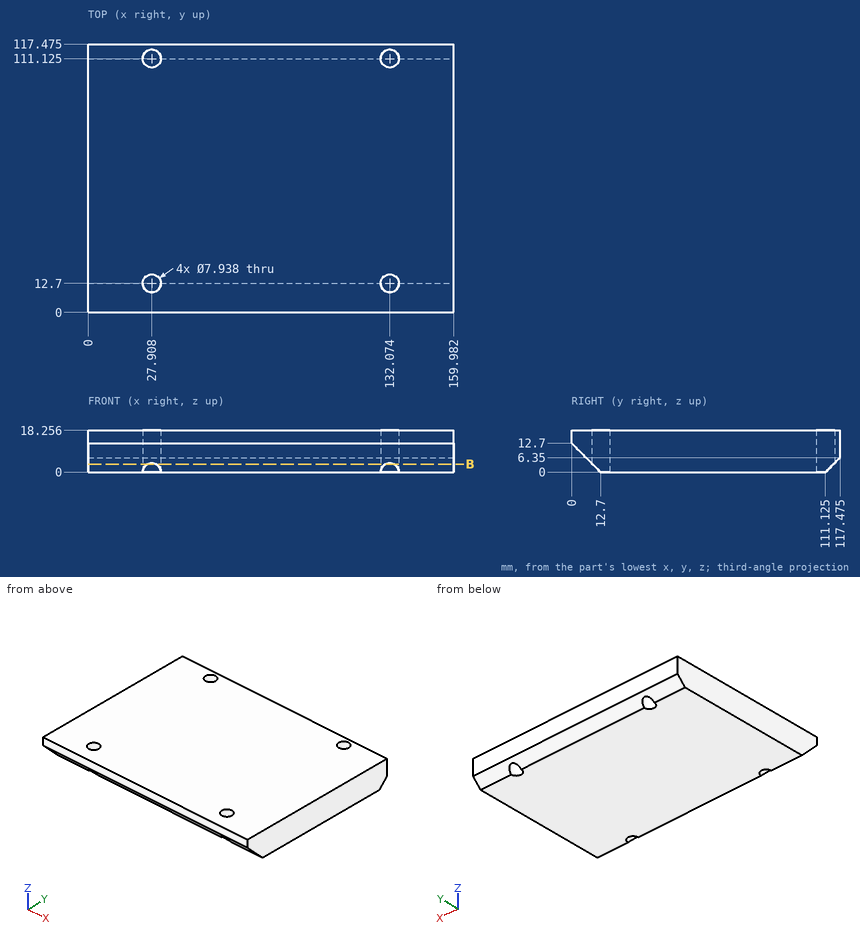
For this review, use the dimensioned drawing (mm, ordinates from the lowest corner) and the shaded views. Give positions to 0.01 mm unless a question says otherwise; leave off trailing zeros. Write each loop counter-clockwise with the first axis right and the second up, starting at its lowest first coordinate (ties: lowest second). Pieces come first, ordered by that corner, then holes.
(1) To check wall thickness, follow L1, parallel to Z at x = 15, y = 5 (1 decimal); L2, parallel to Y at x = 64.5, z = 7.5 (1 decimal); L3, parallel to Y at x = 58, z = 5 (1 decimal). State the ranges of each line that lie inside material, in increasing order.
(2) Consider section B-B, the plane z = 3.5. Give the boundary of the cut face in (x, y) (1 decimal).
(3) For P1, Ø1, axis at x = 45, z = 5, coming from the -Y side; P2, Ø3, axis at x = 125.5, z = 10, coming from the -Y side, all flat-tipped, find the tip position at first contact; note any pin that passes through.
Returned:
1. L1: z = 7.7 to 18.3
1. L2: y = 5.2 to 117.5
1. L3: y = 7.7 to 116.1
2. outline: (0, 9.2) - (26, 9.2) arc R4 cw (long way) to (29.8, 9.2) - (130.2, 9.2) arc R4 cw (long way) to (133.9, 9.2) - (160, 9.2) - (160, 114.6) - (133.9, 114.6) arc R4 cw (long way) to (130.2, 114.6) - (29.8, 114.6) arc R4 cw (long way) to (26, 114.6) - (0, 114.6) - close
3. P1: stops at y = 7.2
3. P2: stops at y = 1.2
